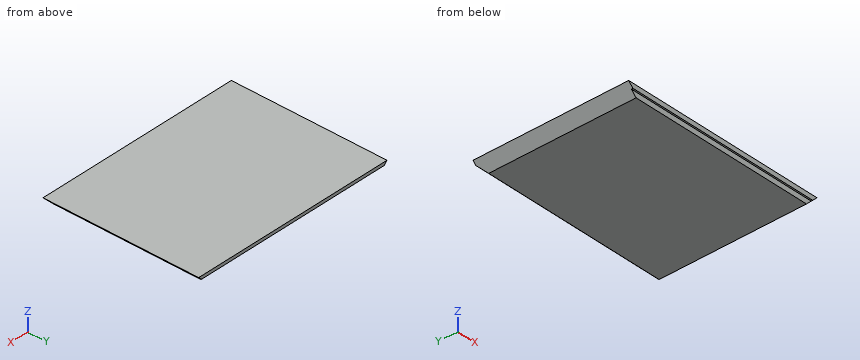
```python
from build123d import *

# Parameters (mm, degrees)
F1_DEPTH = 300
F2_SIZE  = 13
F3_W     = 400
F3_H     = 10
F4_DEPTH = 3


with BuildPart() as f1:
    # F0 (on Front) → F1 (new body)
    with BuildSketch(Plane.XZ):
        Polygon((-19, 19), (0, 0), (362, 0), (381, 19), align=None)
    extrude(amount=F1_DEPTH)

    # F2
    f2_edges = [f1.edges().sort_by_distance(p)[0] for p in [
        (181, 0, 0),
    ]]
    chamfer(f2_edges, length=F2_SIZE)

    # F3 (on face) → F4 (cut)
    with BuildSketch(Plane.XZ.offset(300)):
        with Locations((180, 5)):
            Rectangle(F3_W, F3_H)
    extrude(amount=-F4_DEPTH, mode=Mode.SUBTRACT)


solid = f1.part
```
Could you check a few things on this model? Use its own coordinates, in mm. Coordinates: 2 decimals unless noted, no trailing zeros. Order: outer loops, then holes, each group sorted by start corner. A loop starts at its lowest first (then second) coordinate and runs counter-clockwise, first axis right, second up. Notation, with made-up numbers: M -35.5,-4 L -7.5,-4 A29 ccw -7.5,23 Z; hole C -9,42 d4. An arc over 180 degrees is marked long. Use a Markdown table: item, result. Add a question column.
Q1. I'm going to push flat-ended pins straight in: pin 1 (1.5 mm diameter, centred on y = -109.5, z = 10.5, fed in from +X); pin 2 (2.5 mm diameter, centred on x = 210, y = -298.5, fed in from -Z); pin 3 (5 mm diameter, centred on x = 98, z = 5.5, fed in from -Y). Where does each tip first touch, or does it pass through?
Q2. I want a section at C-C on z = 7. List the corners of the cut face in (x, y) for me.
Q3. I want a section at A-A on x = 154. List the corners of the cut face in (y, z) for me, then the cut area to 3 significant figures.
Q4. I want a section at B-B on y = -174. List the corners of the cut face in (x, z) for me.
Q5. If I drill on L1, parallel to X at y = -228, z = 13; L2, parallel to Y at x = 66.5, z = 12.5; L3, parallel to Y at x = 337, z = 5.75, over which ranges is the centre line in solid material (lowest first)?
Checked values:
| question | item | result |
|---|---|---|
| 1 | pin 1 | x = 373.25 |
| 1 | pin 2 | z = 10 |
| 1 | pin 3 | y = -297 |
| 2 | outline | M -7,-297 L 369,-297 L 369,-6 L -7,-6 Z |
| 3 | outline | M -300,10 L -297,10 L -297,0 L -13,0 L 0,13 L 0,19 L -300,19 Z |
| 3 | area | 5,590 mm² |
| 4 | outline | M -19,19 L 0,0 L 362,0 L 381,19 Z |
| 5 | L1 | -13 to 375 |
| 5 | L2 | -300 to -0.5 |
| 5 | L3 | -297 to -7.25 |
